```python
from build123d import *

# Parameters (mm, degrees)
CROQUIS1_R               = 1.55
CROQUIS1_R_2             = 9.5
SALIENTE_EXTRUIR10_DEPTH = 3
CORTAR_EXTRUIR2_START    = -3
CORTAR_EXTRUIR2_DEPTH    = 3
REDONDEO1_R              = 6
REDONDEO2_R              = 3


# Read off the part's stored shape, not the designer's step: Cortar-Extruir2
with BuildPart() as part:
    # Croquis1 → Saliente-Extruir10 (new body)
    with BuildSketch(Plane(origin=(0, 0, 0), x_dir=(1, 0, 0), z_dir=(0, 1, 0))):
        Polygon((0, 0), (0, 38.7), (10, 38.7), (10, 42), (0, 42), (0, 72), (69.3, 72), (75.3, 72), (75.3, 52), (75.3, 42), (69.3, 42), (69.3, 51.7), (66, 51.7), (66, 42), (50, 42), (50, 38.7), (69.3, 38.7), (69.3, 0), (69.3, -9), (0, -9), align=None)
        with Locations(Location((30, 40.2, 0), (0, 0, 270))):
            Circle(CROQUIS1_R, mode=Mode.SUBTRACT)
        with Locations(Location((67.8, 61.7, 0), (0, 0, 270))):
            Circle(CROQUIS1_R, mode=Mode.SUBTRACT)
        with Locations(Location((29.68, 3.2, 0), (0, 0, 270))):
            Circle(CROQUIS1_R_2, mode=Mode.SUBTRACT)
    extrude(amount=SALIENTE_EXTRUIR10_DEPTH)

    # Cortar-Extruir2 outline → Cortar-Extruir2 (cut)
    with BuildSketch(Plane(origin=(0, 3, 0), x_dir=(1, 0, 0), z_dir=(0, 1, 0)).offset(CORTAR_EXTRUIR2_START)):
        with BuildLine():
            ThreePointArc((26.080222229, -9), (19.492076432, -4.416075983), (16.96, 3.2))
            ThreePointArc((16.96, 3.2), (12.363945378, 19.139693097), (0, 30.2))
            Line((0, 30.2), (0, -9))
            Line((0, -9), (26.080222229, -9))
        make_face()
        with BuildLine():
            ThreePointArc((42.4, 3.2), (39.867923568, -4.416075983), (33.279777771, -9))
            Line((33.279777771, -9), (69.3, -9))
            Line((69.3, -9), (69.3, 30.2))
            ThreePointArc((69.3, 30.2), (51.011487425, 21.520592158), (42.4, 3.2))
        make_face()
        with BuildLine():
            Line((0, 72), (0, 45))
            ThreePointArc((0, 45), (34.270978976, 52.034382388), (63, 72))
            Line((63, 72), (0, 72))
        make_face()
    extrude(amount=CORTAR_EXTRUIR2_DEPTH, mode=Mode.SUBTRACT)

    # Redondeo1
    redondeo1_edges = [part.edges().sort_by_distance(p)[0] for p in [
        (75.3, 1.5, -72),
    ]]
    fillet(redondeo1_edges, radius=REDONDEO1_R)

    # Redondeo2
    redondeo2_edges = [part.edges().sort_by_distance(p)[0] for p in [
        (69.3, 1.5, -30.2),
        (0, 1.5, -45),
        (0, 1.5, -30.2),
    ]]
    fillet(redondeo2_edges, radius=REDONDEO2_R)


solid = part.part
```
The model under review builds one solid part; all positions refer to its coordinate system, in mm. A direction names the side the tool comes from. Give positions to 0.01 mm unless a question says otherwise; leave off trailing zeros. Write each loop counter-clockwise with the first axis right and the second up, starting at its lowest first coordinate (ties: lowest second). Pieces come first, ordered by that corner, then holes.
(1) Tool access review of faces 4 (the cylindrical face through (12.93, 1.48, -18.2)), 5 (the flat face through (69.3, 1, -47)), 6 (the flat face through (50, 1, -40)), 7 (the flat face through (69.3, 1, -36)), 8 (the flat face through (10, 1, -40)): name each direction out of +Z, -Z, +X, -X, +Y, -Y from which nothing blocks a thin tool from reaching the whole face with its end or side.
(2) Consider section D-D, the plane z = 3.5. Give the boundary of the cut face in (x, y), and give its area (3 significant figures).
(3) The part is to be moulded in two halves that separate along X. For faces 1 (the cylindrical face through (67.206, 1.479, -60.268)), 2 (the cylindrical face through (19.561, 1.479, 4.507)), 3 (the cylindrical face through (73.589, 1.521, -70.196)), say which applies: released by +X, released by -X, zero draft, split by the parting line, or undercut.
(4) For P1, Ø0.9, axis at x = 6, y = 1.5, coming from the +Z side; P2, Ø1, axis at y = 1.5, z = -11, coming from the +X side; P3, Ø1.5, axis at y = 1.5, z = -41, coming from the -X side; P4, Ø1.9, axis at x = 30, z = -40.2, coming from the +Y side, all flat-tipped, find the tip position at first contact; note any pin that passes through.
(5) Consider section C-C, the plane x = 67.8. Give the boundary of the cut face in (y, z).
(6) Consider section B-B, the plane z = -10. Give the boundary of the cut face in (x, y), and give its area (3 significant figures).
(7) To check wall thickness, follow L1, parallel to X at y = 1.2, z = -40.2; L2, parallel to Z at x = 67.8, y = 2.25; L3, parallel to Z at x = 33, y = 2.65. State the ranges of each line that lie inside material, in increasing order.
(8) Consider section A-A, the plane y = 2.2. Give the boundary of the cut face in (x, z).
Returned:
1. face 4: +Z, -X, +Y, -Y
1. face 5: +Y, -Y
1. face 6: +X, +Y, -Y
1. face 7: +Z, +X, +Y, -Y
1. face 8: -X, +Y, -Y
2. outline: (18.87, 0) - (22.95, 0) - (22.95, 3) - (18.87, 3) - close; (36.41, 0) - (40.49, 0) - (40.49, 3) - (36.41, 3) - close
2. area: 24.5 mm2
3. face 1: undercut
3. face 2: released by -X
3. face 3: released by +X
4. P1: stops at z = -25.99
4. P2: stops at x = 44.41
4. P3: stops at x = 10
4. P4: passes through
5. outline: (0, -72) - (3, -72) - (3, -63.25) - (0, -63.25) - close; (0, -60.15) - (3, -60.15) - (3, -51.7) - (0, -51.7) - close; (0, -38.7) - (3, -38.7) - (3, -30.21) - (0, -30.21) - close
6. outline: (16.18, 0) - (23.05, 0) - (23.05, 3) - (16.18, 3) - close; (36.31, 0) - (43.86, 0) - (43.86, 3) - (36.31, 3) - close
6. area: 43.2 mm2
7. L1: x = 10 to 28.45, 31.55 to 50
7. L2: z = -72 to -63.25, -60.15 to -51.7, -38.7 to -30.21
7. L3: z = -51.5 to -12.1, 5.7 to 9
8. outline: (0, -42.05) arc R3 ccw to (2.9, -45.05) arc R87 cw to (63, -72) - (69.3, -72) arc R6 ccw to (75.3, -66) - (75.3, -42) - (69.3, -42) - (69.3, -51.7) - (66, -51.7) - (66, -42) - (50, -42) - (50, -38.7) - (69.3, -38.7) - (69.3, -32.8) arc R3 ccw to (66.84, -29.85) arc R30 cw to (42.4, -3.2) arc R12.72 ccw to (33.28, 9) - (26.08, 9) arc R12.72 ccw to (16.96, -3.2) arc R30 cw to (1.54, -29.4) arc R3 ccw to (0, -32.02) - (0, -38.7) - (10, -38.7) - (10, -42) - (0, -42) - close; hole circle Ø19 at (29.68, -3.2); hole circle Ø3.1 at (30, -40.2); hole circle Ø3.1 at (67.8, -61.7)
